from build123d import *

# Parameters (mm, degrees)
F0_W     = 35.56
F0_H     = 35.56
F1_DEPTH = 5.08
F2_W     = 19.812
F2_H     = 4.572
F3_DEPTH = 2.54
F4_W     = 19.812
F4_H     = 4.572
F5_DEPTH = 2.54
F6_W     = 20.32
F6_H     = 5.08
F7_DEPTH = 2.54
F8_W     = 20.32
F8_H     = 5.08
F9_DEPTH = 2.54


with BuildPart() as f1:
    # F0 (on Top) → F1 (new body, symmetric)
    with BuildSketch(Plane.XY):
        Rectangle(F0_W, F0_H)
        with BuildLine():
            Line((5.3660807292, 12.4850260417), (10.6908203125, 12.4850260417))
            Line((10.6908203125, 12.4850260417), (10.6908203125, -3.8088975694))
            add(Edge.make_bspline(
                [(10.6908203125, -3.8088975694), (10.6908203125, -6.6035590278), (9.4423177083, -8.7036892361)],
                knots=[0, 0, 0, 1, 1, 1], degree=2))
            add(Edge.make_bspline(
                [(9.4423177083, -8.7036892361), (8.1938151042, -10.8038194444), (5.8318576389, -11.9255425347)],
                knots=[0, 0, 0, 1, 1, 1], degree=2))
            add(Edge.make_bspline(
                [(5.8318576389, -11.9255425347), (3.4699001736, -13.047265625), (0.2508029514, -13.047265625)],
                knots=[0, 0, 0, 1, 1, 1], degree=2))
            add(Edge.make_bspline(
                [(0.2508029514, -13.047265625), (-4.6054036458, -13.047265625), (-7.292578125, -10.5557725694)],
                knots=[0, 0, 0, 1, 1, 1], degree=2))
            add(Edge.make_bspline(
                [(-7.292578125, -10.5557725694), (-9.9797526042, -8.0642795139), (-9.9797526042, -3.7427517361)],
                knots=[0, 0, 0, 1, 1, 1], degree=2))
            Line((-9.9797526042, -3.7427517361), (-9.9797526042, 12.4850260417))
            Line((-9.9797526042, 12.4850260417), (-4.6605251736, 12.4850260417))
            Line((-4.6605251736, 12.4850260417), (-4.6605251736, -2.9324652778))
            add(Edge.make_bspline(
                [(-4.6605251736, -2.9324652778), (-4.6605251736, -5.8428819444), (-3.4891927083, -7.2043836806)],
                knots=[0, 0, 0, 1, 1, 1], degree=2))
            add(Edge.make_bspline(
                [(-3.4891927083, -7.2043836806), (-2.3178602431, -8.5658854167), (0.3886067708, -8.5658854167)],
                knots=[0, 0, 0, 1, 1, 1], degree=2))
            add(Edge.make_bspline(
                [(0.3886067708, -8.5658854167), (3.0068793403, -8.5658854167), (4.1864800347, -7.1961154514)],
                knots=[0, 0, 0, 1, 1, 1], degree=2))
            add(Edge.make_bspline(
                [(4.1864800347, -7.1961154514), (5.3660807292, -5.8263454861), (5.3660807292, -2.8993923611)],
                knots=[0, 0, 0, 1, 1, 1], degree=2))
            Line((5.3660807292, -2.8993923611), (5.3660807292, 12.4850260417))
        make_face(mode=Mode.SUBTRACT)
    extrude(amount=F1_DEPTH, both=True)

    # F2 (on face) → F3 (join)
    with BuildSketch(Plane(origin=(0, 17.78, 0), x_dir=(-1, 0, 0), z_dir=(0, 1, 0))):
        Rectangle(F2_W, F2_H)
    extrude(amount=F3_DEPTH)

    # F4 (on face) → F5 (join)
    with BuildSketch(Plane(origin=(-17.78, 0, 0), x_dir=(0, -1, 0), z_dir=(-1, 0, 0))):
        Rectangle(F4_W, F4_H)
    extrude(amount=F5_DEPTH)

    # F6 (on face) → F7 (cut)
    with BuildSketch(Plane.XZ.offset(17.78)):
        Rectangle(F6_W, F6_H)
    extrude(amount=-F7_DEPTH, mode=Mode.SUBTRACT)

    # F8 (on face) → F9 (cut)
    with BuildSketch(Plane.YZ.offset(17.78)):
        Rectangle(F8_W, F8_H)
    extrude(amount=-F9_DEPTH, mode=Mode.SUBTRACT)


solid = f1.part
Source: CAD feature listing. Evaluate the final solid. Frame: model axes, mm. A direction names the side the tool comes from. Give positions to 0.01 mm unless a question says otherwise; leave off trailing zeros. Write each loop counter-clockwise with the first axis right and the second up, starting at its lowest first coordinate (ties: lowest second). Pieces come first, ordered by that corner, then holes. Notation, with made-up numbers: M 65,66.5 L 94,66.5 A16 cw 94,80.5 Z; hole C -34,40.5 d2. An arc over 180 degrees is marked long. Return JSON: item names as keys, results as strings. Group by question number.
1) Cut plane A-A, the plane y = 9. Output: boundary loops of the cut face in (x, z).
2) Ray query, L1, parallel to X at y = 1, z = 4.25; L2, parallel to X at y = 1.5, z = 1.5; L3, parallel to Y at x = 15.5, z = -0.75. Return the intervals inside material, ascending.
3) Set-up query: faces 1 (the face through (5.366, 5, 0)), 2 (the face through (17, 10.16, 0)), 3 (the face through (-19, 0, -2.286)), 4 (the face through (0, 19, 2.286)). Return all of +Z, -Z, +X, -X, +Y, -Y with unobstructed straight access to the full face (end or side cutting, diameter ignored); none if empty.
4) Draft query along X for faces 5 (the face through (17.78, 0, 3)), 6 (the face through (0, -15.24, 0)), 7 (the face through (0, 0, -5.08)), 8 (the face through (0, -17, 2.54)). Return one class per face: released by +X, released by -X, zero draft, split by the parting line, or undercut.
5) Cut plane B-B, the plane y = -14.5. Output: boundary loops of the cut face in (x, z), then the cut area to 3 significant figures.
6) Cut plane D-D, the plane y = -6.5. Give the number of separate pieces and of enclosed holes in the cut face, then the cut area to 3 significant figures.
7) First-contact query: pin 1 Ø1.6 at (x, z) = (-8.5, -1.5) entering from -Y; pin 2 Ø0.8 at (x, y) = (4, 19.5) entering from +Z; pin 3 Ø2 at (y, z) = (7.5, 0) entering from +X; pin 4 Ø1.5 at (x, y) = (0.5, -9.5) entering from -Z. Flat tips, straight axial feed; report the tip coordinate or a pass-through.
Data:
{
 "1": {"outline": "M -20.32,-2.29 L -17.78,-2.29 L -17.78,-5.08 L -9.98,-5.08 L -9.98,5.08 L -17.78,5.08 L -17.78,2.29 L -20.32,2.29 Z; M -4.66,-5.08 L 5.37,-5.08 L 5.37,5.08 L -4.66,5.08 Z; M 10.69,-5.08 L 17.78,-5.08 L 17.78,-2.54 L 15.24,-2.54 L 15.24,2.54 L 17.78,2.54 L 17.78,5.08 L 10.69,5.08 Z"},
 "2": {"L1": "x = -17.78 to -9.98, -4.66 to 5.37, 10.69 to 17.78", "L2": "x = -20.32 to -9.98, -4.66 to 5.37, 10.69 to 15.24", "L3": "y = -17.78 to -10.16, 10.16 to 17.78"},
 "3": {"face 1": "+Z, -Z", "face 2": "+X", "face 3": "-Z, -X, +Y, -Y", "face 4": "+Z, +X, -X, +Y"},
 "4": {"face 5": "released by +X", "face 6": "undercut", "face 7": "zero draft", "face 8": "undercut"},
 "5": {"outline": "M -17.78,-5.08 L 17.78,-5.08 L 17.78,5.08 L -17.78,5.08 Z", "area": "361 mm²"},
 "6": {"separate pieces": "3", "enclosed holes": "0", "area": "244 mm²"},
 "7": {"pin 1": "stops at y = -15.24", "pin 2": "stops at z = 2.29", "pin 3": "stops at x = 15.24", "pin 4": "passes through"}
}
